Design review of the part built by this model. Coordinates are the model's own, in mm. A direction names the side the tool comes from. Round coordinates to 2 decimals unless told otherwise and drop trailing zeros. Order: outer loops, then holes, each group sorted by start corner. A loop starts at its lowest first (then second) coordinate and runs counter-clockwise, first axis right, second up. Notation, with made-up numbers: M 45.25,-28 L 77.25,-28 A27 ccw 77.25,-10 Z; hole C -15.5,57 d4. An arc over 180 degrees is marked long. Use a Markdown table: item, result. Add a question column.
(1) To check wall thickness, follow probe 1 along Z at (x, y) = (-36, 10); probe 2 along Y at (x, z) = (-27, -55); probe 3 along Y at (x, z) = (-32, -130). State the ranges of each line that lie inside material, in increasing order. Write a range as from..to.
(2) Take a section at A-A (z = -78.5). Write out the cut boundary in (x, y), then the cut area to 3 significant figures.
(3) Machinability: for faces 1 (the face through (-36.866, -12.888, -101.372)), 2 (the face through (-27, 60.593, -101)), which of the approach directions +Z, -Z, +X, -X, +Y, -Y give a long, thin tool a straight path to every point of the face, cutting with its end or side? Answer none if there is none.
(4) For pin 1 (5 mm diameter, centred on x = -46.5, z = -27.5, fed in from -Y); pin 2 (1.5 mm diameter, centred on x = -36, z = -177.5, fed in from +Y); pin 3 (12 mm diameter, centred on x = -27, z = -122, fed in from -Y), all flat-tipped, find the tip position at first contact; note any pin that passes through.
(5) The part is to be moulded in two halves that separate along Y. For faces 3 (the face through (-36.6, -10.89, -101.37)), 4 (the face through (-36.25, -12.46, -0.6)), 5 (the face through (-27, 62.593, -101)), 6 (the face through (-33, 23, -2)), say which applies: released by +Y, released by -Y, zero draft, split by the parting line, or undercut.
```python
from build123d import *

# Parameters (mm, degrees)
FILLET2_R    = 2
SHELL2_START = -198
SHELL2_DEPTH = 196


# Read off the part's stored shape, not the designer's step: Shell2
with BuildPart() as part:
    # Sweep2: sweep along a path in Sketch6
    with BuildLine(Plane(origin=(0, 62.593086106, 0), x_dir=(1, 0, 0), z_dir=(0, 1, 0))) as sweep2_path:
        Line((-20, 0), (-20, 200))
    # Sketch5 → Sweep2 (sweep)
    with BuildSketch(Plane.XY):
        Polygon((-20, -17.406913894), (-20, 62.593086106), (-35, 62.593086106), (-55.232597818, -7.966367761), align=None)
    sweep(path=sweep2_path.line)

    # Fillet2
    fillet2_edges = [part.edges().sort_by_distance(p)[0] for p in [
        (-27.5, 62.593086106, 0),
        (-45.116298909, 27.313359172, 0),
        (-55.232597818, -7.966367761, -100),
        (-37.616298909, -12.686640828, -200),
        (-27.5, 62.593086106, -200),
        (-35, 62.593086106, -100),
        (-45.116298909, 27.313359172, -200),
        (-37.616298909, -12.686640828, 0),
    ]]
    fillet(fillet2_edges, radius=FILLET2_R)

    # Shell2 outline → Shell2 (cut)
    with BuildSketch(Plane.XY.offset(SHELL2_START)):
        Polygon((-52.749093204, -6.561268456), (-20, -15.336361533), (-20, 60.593086106), (-33.4928919, 60.593086106), align=None)
    extrude(amount=SHELL2_DEPTH, mode=Mode.SUBTRACT)


solid = part.part
```
Verdict:
| question | item | result |
|---|---|---|
| 1 | probe 1 | z = -200..-198, -2..0 |
| 1 | probe 2 | y = -15.53..-13.46, 60.59..62.59 |
| 1 | probe 3 | y = -14.19..-12.12, 60.59..62.59 |
| 2 | outline | M -54.67,-6.01 A2 ccw -53.27,-8.49 L -20,-17.41 L -20,-15.34 L -52.75,-6.56 L -33.49,60.59 L -20,60.59 L -20,62.59 L -33.49,62.59 A2 ccw -35.42,61.14 Z |
| 2 | area | 241 mm^2 |
| 3 | face 1 | +Z, -Z, -X, -Y |
| 3 | face 2 | +X |
| 4 | pin 1 | stops at y = -10.98 |
| 4 | pin 2 | stops at y = 61.55 |
| 4 | pin 3 | stops at y = -17.14 |
| 5 | face 3 | undercut |
| 5 | face 4 | released by -Y |
| 5 | face 5 | released by +Y |
| 5 | face 6 | undercut |
